from build123d import *

# Parameters (mm, degrees)
ESQUISSE1_W             = 13.5
ESQUISSE1_H             = 29
ESQUISSE2_R             = 11.5
ENL_V_MAT_EXTRU_1_DEPTH = 4
CHANFREIN1_SIZE         = 1
ESQUISSE4_R             = 8
ENL_V_MAT_EXTRU_2_DEPTH = 10
ESQUISSE5_R             = 5
ENL_V_MAT_EXTRU_3_DEPTH = 25.279621196
ENL_V_MAT_EXTRU_4_REACH = 43.033
ESQUISSE6_R             = 3


with BuildPart() as part:
    # Esquisse1 → Base-Révolution (revolve)
    with BuildSketch(Plane.XY, mode=Mode.PRIVATE) as base_r_volution_sk:
        with Locations((6.75, 14.5)):
            Rectangle(ESQUISSE1_W, ESQUISSE1_H)
    revolve(base_r_volution_sk.sketch.rotate(Axis((0, 0, 0), (0, 1, 0)), 90), axis=Axis((0, 0, 0), (0, 1, 0)))

    # Esquisse2 → Enlèv. mat.-Extru.1 (cut)
    with BuildSketch(Plane.XZ):
        with Locations(Location((0, 0, 0), (0, 0, 270))):
            Circle(ESQUISSE2_R)
    extrude(amount=-ENL_V_MAT_EXTRU_1_DEPTH, mode=Mode.SUBTRACT)

    # Chanfrein1
    chanfrein1_edges = [part.edges().sort_by_distance(p)[0] for p in [
        (0, 0, 13.5),
        (0, 29, 13.5),
    ]]
    chamfer(chanfrein1_edges, length=CHANFREIN1_SIZE)

    # Esquisse3 → Enlèvement de matière-Révolution1 (revolve, cut)
    with BuildSketch(Plane(origin=(0, 0, 0), x_dir=(1, 0, 0), z_dir=(0, 1, 0))):
        Polygon((0, 12.2), (16.5, 12.2), (21.5, 17.2), (0, 17.2), align=None)
    revolve(axis=Axis((0, 0, 0), (0, 0, -1)), mode=Mode.SUBTRACT)

    # Esquisse4 → Enlèv. mat.-Extru.2 (cut)
    with BuildSketch(Plane.XZ.offset(-4)):
        with Locations(Location((0, 0, 0), (0, 0, 270))):
            Circle(ESQUISSE4_R)
    extrude(amount=-ENL_V_MAT_EXTRU_2_DEPTH, mode=Mode.SUBTRACT)

    # Esquisse5 → Enlèv. mat.-Extru.3 (cut, through all)
    with BuildSketch(Plane.XZ.offset(-14)):
        with Locations(Location((0, 0, 0), (0, 0, 270))):
            Circle(ESQUISSE5_R)
    extrude(amount=-ENL_V_MAT_EXTRU_3_DEPTH, mode=Mode.SUBTRACT)

    # Esquisse6 → Enlèv. mat.-Extru.4 (cut, up to next)
    with BuildSketch(Plane(origin=(0, 0, -12.2), x_dir=(-1, 0, 0), z_dir=(0, 0, -1)), mode=Mode.PRIVATE) as enl_v_mat_extru_4_sk1:
        with Locations((0, 8)):
            Circle(ESQUISSE6_R)
    enl_v_mat_extru_4_tool1 = extrude(enl_v_mat_extru_4_sk1.sketch, amount=-ENL_V_MAT_EXTRU_4_REACH, mode=Mode.PRIVATE) & part.part
    add(enl_v_mat_extru_4_tool1.solids().sort_by_distance((0, 8, -12.2))[0], mode=Mode.SUBTRACT)


solid = part.part
For this review, take the finished solid that the model builds, in its own axes (mm). A direction names the side the tool comes from. Give positions to 0.01 mm unless a question says otherwise; leave off trailing zeros. Write each loop counter-clockwise with the first axis right and the second up, starting at its lowest first coordinate (ties: lowest second). Pieces come first, ordered by that corner, then holes. Notation, with made-up numbers: (24, 87) -> (77, 87) arc R31 cw to (77, 116) -> close; hole circle Ø8 at (-11.75, 8.25). An arc over 180 degrees is marked (long way). Use CSV: the item, a comma, the result in double quotes.
Q1. Take a section at A-A, the plane x = 0. Write out the cut boundary in (y, z).
Conclusion:
outline,"(0, -12.2) -> (5, -12.2) -> (5, -8) -> (4, -8) -> (4, -11.5) -> (0, -11.5) -> close; (0, 11.5) -> (4, 11.5) -> (4, 8) -> (14, 8) -> (14, 5) -> (29, 5) -> (29, 12.5) -> (28, 13.5) -> (1, 13.5) -> (0, 12.5) -> close; (11, -12.2) -> (16.5, -12.2) -> (17.8, -13.5) -> (28, -13.5) -> (29, -12.5) -> (29, -5) -> (14, -5) -> (14, -8) -> (11, -8) -> close"
Q2. Mouldability with a two-part tool opening along Z and no side actions: class faces 4 (the face through (-4.868, 8.93, 6.349)), 5 (the face through (3, 10, -12.2)), 6 (the face through (-4.88, 21.4, 1.08)), 7 (the face through (-0.594, 14.689, 13.487)) as pulls with the +Z half, pulls with the -Z half, needs draft (parallel to the pull), parting line crosses it, or undercut.
Conclusion:
face 4,"undercut"
face 5,"pulls with the -Z half"
face 6,"undercut"
face 7,"parting line crosses it"
Q3. For P1, Ø6, axis at x = 1, y = 8.5, coming from the -Z side; P2, Ø1, axis at y = 3.5, z = 7.5, coming from the +X side; P3, Ø6, axis at y = 10, z = -4.5, coming from the +X side; P4, Ø9, axis at x = 0, z = 0, coming from the +Y side, all flat-tipped, find the tip position at first contact; note any pin that passes through.
Conclusion:
P1,"z = -12.2"
P2,"x = 11.54"
P3,"x = 13.42"
P4,"through"
Q4. Tool access review of faces 1 (the face through (3, 8, -10)), 2 (the face through (-0.1, 16.9, -12.6)), 3 (the face through (8, 4, -2)): name each direction out of +Z, -Z, +X, -X, +Y, -Y from which nothing blocks a thin tool from reaching the whole face with its end or side.
Conclusion:
face 1,"-Z"
face 2,"-Z, -Y"
face 3,"-Y"
Q5. Take a section at D-D, the plane y = 13.5. Write out the cut boundary in (x, z).
Conclusion:
outline,"(-5.78, -12.2) -> (5.78, -12.2) arc R13.5 ccw (long way) to start; hole circle Ø16 at (0, 0)"
Q6. Take a section at C-C, the plane y = 8. Write out the cut boundary in (x, z).
Conclusion:
outline,"(-5.78, -12.2) -> (-3, -12.2) -> (-3, -7.42) arc R8 cw (long way) to (3, -7.42) -> (3, -12.2) -> (5.78, -12.2) arc R13.5 ccw (long way) to start"
Q7. Take a section at B-B, the plane z = 0. Write out the cut boundary in (x, y).
Conclusion:
outline,"(-13.5, 1) -> (-12.5, 0) -> (-11.5, 0) -> (-11.5, 4) -> (-8, 4) -> (-8, 14) -> (-5, 14) -> (-5, 29) -> (-12.5, 29) -> (-13.5, 28) -> close; (5, 14) -> (8, 14) -> (8, 4) -> (11.5, 4) -> (11.5, 0) -> (12.5, 0) -> (13.5, 1) -> (13.5, 28) -> (12.5, 29) -> (5, 29) -> close"
Q8. To check wall thickness, follow probe 1 along X at (y, z) = (11, 0); probe 2 along X at (y, z) = (19, 0); probe 3 along Y at (x, z) = (0, -11). State the ranges of each line that lie inside material, in increasing order. Write a range as [from, to].
Conclusion:
probe 1,"[-13.5, -8], [8, 13.5]"
probe 2,"[-13.5, -5], [5, 13.5]"
probe 3,"[4, 5], [11, 29]"
